Answer from the drawing. Dimensions are ordinates in mm from the lowest x, y and z of the part. A direction names the side the tool comes from. Give positions to 0.01 mm unless a question says otherwise; leave off trailing zeros. Loops run counter-clockwise (first coordinate to the right, second up) from the corner with the lowest first, then second, coordinate; pieces in that order, holes last. Notation, with made-up numbers: (27.5, 5) - (76.5, 5) arc R24 ccw to (76.5, 17) - close; hole circle Ø11 at (-33, 16). An arc over 180 degrees is marked (long way). One line per item, written item: value.
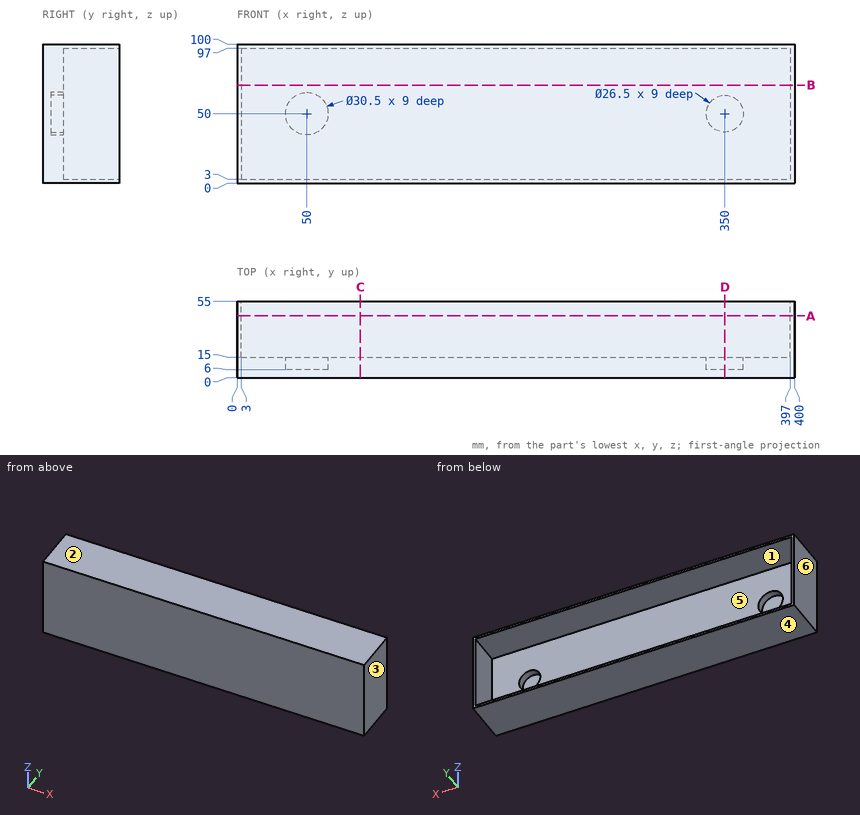
1. The mould has two halves that part along Z. Classify the marked faces 1, 2, 3 and 4: released by +Z, released by -Z, zero draft, split by the parting line, or undercut.
Output:
face 1: undercut
face 2: released by +Z
face 3: zero draft
face 4: released by -Z
2. Section A-A (y = 44.5) is taken. Write down the section's boundary in (x, z), and give its area (3 significant figures).
Output:
outline: (0, 0) - (400, 0) - (400, 100) - (0, 100) - close; hole (3, 3) - (397, 3) - (397, 97) - (3, 97) - close
area: 2,960 mm²
3. Section D-D (x = 350) is taken. Write down the section's boundary in (y, z), and give its area (3 significant figures).
Output:
outline: (0, 0) - (55, 0) - (55, 3) - (15, 3) - (15, 36.75) - (6, 36.75) - (6, 63.25) - (15, 63.25) - (15, 97) - (55, 97) - (55, 100) - (0, 100) - close
area: 1,500 mm²
4. For the marked faces 5 and 6, determine the directions among +Z, -Z, +X, -X, +Y, -Y from which every point of the face is accessible in a straight line to the end or side of a thin tool.
Output:
face 5: +Y
face 6: +Z, -Z, -X, +Y, -Y
5. Flat-ended cylindrical pins translate along their axes: pin 1 Ø3 at (x, z) = (345.5, 59.5) entering from -Y; pin 2 Ø2 at (x, z) = (102, 46) entering from +Y; pin 3 Ø18.5 at (x, z) = (50, 50) entering from +Y. Find the tip coordinate at first contact, or state that the pin passes through.
Output:
pin 1: stops at y = 0
pin 2: stops at y = 15
pin 3: stops at y = 6
6. Section C-C (x = 88.5) is taken. Write down the section's boundary in (y, z), and give its area (3 significant figures).
Output:
outline: (0, 0) - (55, 0) - (55, 3) - (15, 3) - (15, 97) - (55, 97) - (55, 100) - (0, 100) - close
area: 1,740 mm²
7. Section B-B (z = 70.5) is taken. Write down the section's boundary in (x, y), and give its area (3 significant figures).
Output:
outline: (0, 0) - (400, 0) - (400, 55) - (397, 55) - (397, 15) - (3, 15) - (3, 55) - (0, 55) - close
area: 6,240 mm²
8. Find the intervals of material crossed by line 1 along X through (y, z) = (9, 50); line 2 along X through (y, z) = (49.5, 14); line 3 along Z through (x, y) = (296.5, 45.5), in increasing order.
Output:
line 1: x = 0 to 34.75, 65.25 to 336.75, 363.25 to 400
line 2: x = 0 to 3, 397 to 400
line 3: z = 0 to 3, 97 to 100
